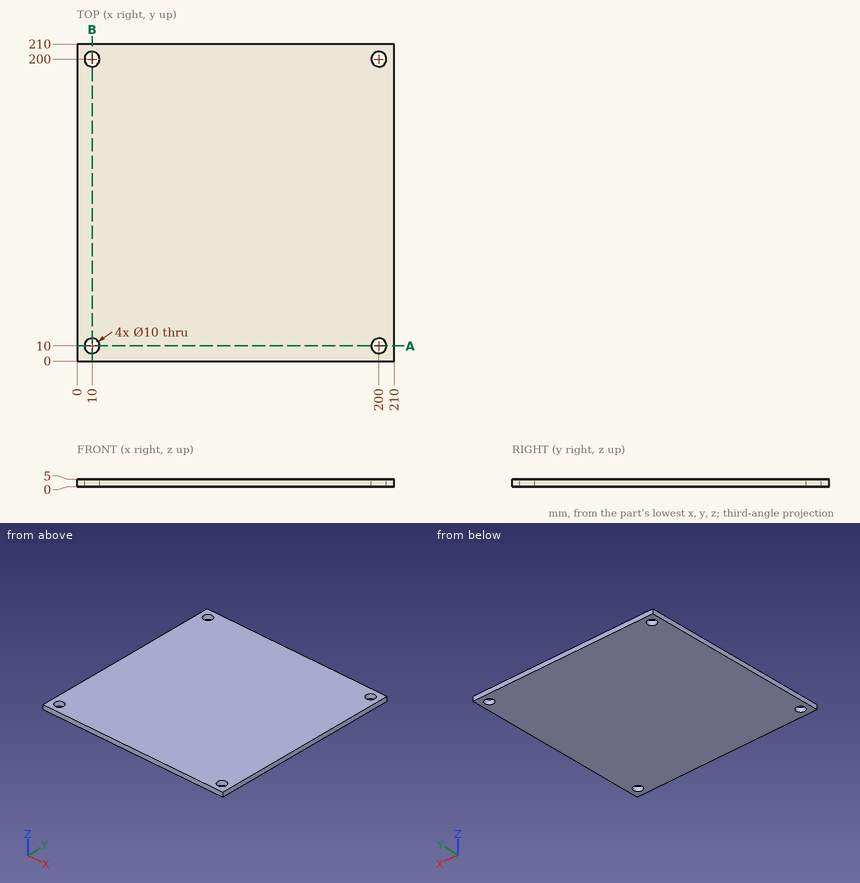
Here's the drawing with two shaded views (mm, measured from the low corner). I have some questions. Give positions to 0.01 mm unless a question says otherwise; leave off trailing zeros. Write each loop counter-clockwise with the first axis right and the second up, starting at its lowest first coordinate (ties: lowest second). Pieces come first, ordered by that corner, then holes. Notation, with made-up numbers: (-15, -16) -> (8, -16) arc R35 ccw to (8, 17) -> close; hole circle Ø7 at (-37, 24). An arc over 180 degrees is marked (long way). One line per item, written item: value.
Q1. For P1, Ø6, axis at x = 10, y = 10, coming from the +Z side, with a flat end and sliding along its axis, tell me the tip position at first contact or that it passes through.
Results found:
P1: passes through
Q2. Imagine slicing it at A-A on y = 10. Please give me the cut outline in (x, z).
Results found:
outline: (0, 0) -> (5, 0) -> (5, 5) -> (0, 5) -> close; (15, 0) -> (195, 0) -> (195, 5) -> (15, 5) -> close; (205, 0) -> (210, 0) -> (210, 5) -> (205, 5) -> close
Q3. Please list where these lines run through material, in increasing order: line 1 (Y direction, x = 200, z = 1.5); line 2 (Y direction, x = 196, z = 4.35). Write a range as [from, to].
Results found:
line 1: y = [0, 5], [15, 195], [205, 210]
line 2: y = [0, 7], [13, 197], [203, 210]
